from build123d import *

# Parameters (mm, degrees)
F1_DEPTH   = 762
F2_W       = 12.7
F2_H       = 25.4
F1_FACE1_W = 762
F1_FACE1_H = 7.0995158286
F3_DEPTH   = 38.101
F5_DEPTH   = 635.001
F7_DEPTH   = 635.001


# Not quite as in the source:
# - a feature names something its author has since deleted; it is built from what else it names


with BuildPart() as f1:
    # F0 (on Right) → F1 (new body)
    with BuildSketch(Plane.YZ):
        Polygon((-76.2, 6.35), (-127, -15.875), (-120.65, -19.05), (127, -19.05), (-25.4, 19.05), align=None)
    extrude(amount=F1_DEPTH)

    # F2 (on face) + F1_face1 (on face) → F3 (cut, through all)
    with BuildSketch(Plane(origin=(0, 0, -19.05), x_dir=(1, 0, 0), z_dir=(0, 0, -1))):
        Polygon((0, 120.65), (0, -127), (76.2, -127), (76.2, -76.2), (381, -76.2), (393.7, -76.2), (406.4, -76.2), (711.2, -76.2), (711.2, -127), (762, -127), (762, 120.65), align=None)
        with Locations((387.35, -88.9)):
            Rectangle(F2_W, F2_H)
        with Locations((400.05, -88.9)):
            Rectangle(F2_W, F2_H)
    with BuildSketch(Plane(origin=(381, -123.825, -17.4625), x_dir=(1, 0, 0), z_dir=(0, -0.4472135955, -0.894427191))):
        Rectangle(F1_FACE1_W, F1_FACE1_H)
    extrude(amount=-F3_DEPTH, dir=(0, 0, -1), mode=Mode.SUBTRACT)

    # F4 (on face) → F5 (cut, through all)
    with BuildSketch(Plane(origin=(76.2, 0, 0), x_dir=(0, -1, 0), z_dir=(-1, 0, 0))):
        Polygon((-76.2, -6.35), (-82.55, -7.9375), (-76.2, -15.875), align=None)
        Polygon((-76.2, -15.875), (-82.55, -19.05), (-76.2, -19.05), align=None)
    extrude(amount=-F5_DEPTH, mode=Mode.SUBTRACT)

    # F6 (on face) → F7 (cut, through all)
    with BuildSketch(Plane(origin=(76.2, 0, 0), x_dir=(0, -1, 0), z_dir=(-1, 0, 0))):
        with BuildLine():
            ThreePointArc((-82.55, -17.4625), (-81.4274679849, -16.9975320151), (-80.9625, -15.875))
            ThreePointArc((-80.9625, -15.875), (-83.6725320151, -14.7524679849), (-82.55, -17.4625))
        make_face()
    extrude(amount=-F7_DEPTH, mode=Mode.SUBTRACT)


solid = f1.part
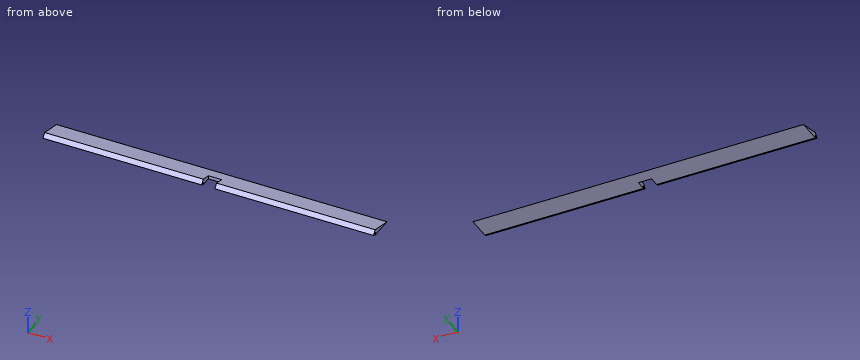
Build history of the part. All positions in model axes, mm. Round coordinates to 2 decimals unless told otherwise and drop trailing zeros. Loops run counter-clockwise (first coordinate to the right, second up) from the corner with the lowest first, then second, coordinate; pieces in that order, holes last. Notation, with made-up numbers: (-22.5, 32) -> (-3.5, 32) arc R10 ccw to (-3.5, 38) -> close; hole circle Ø10 at (-31.75, 44). An arc over 180 degrees is marked (long way). Use CSV: the item, a comma, the result in double quotes. Start each with the question number.
Q1. Flat gauge pins, fed straight in: pin 1 Ø3 at (x, z) = (393, -16.5) entering from -Y; pin 2 Ø5 at (y, z) = (94, -10) entering from +X; pin 3 Ø5 at (x, z) = (199, -12) entering from -Y; pin 4 Ø6 at (x, y) = (607.5, 84.5) entering from +Z. Where does each tip first touch, or does it go through?
Q2. Drill centre lines: L1, parallel to Z at x = 271, y = 83; L2, parallel to X at y = 90, z = -13; L3, parallel to Z at x = 202.5, y = 82.55. Where is each one in solid material? Low to high.
Q3. Saw through at A-A on z = -11. Give the cut face in (x, y), and give its area (3 significant figures).
Q4. Saw through at C-C on y = 113. Give the cut face in (x, z), and give its area (3 significant figures).
Solutions:
1,pin 1,"stops at y = 101.6"
1,pin 2,"stops at x = 711.2"
1,pin 3,"stops at y = 77.3"
1,pin 4,"stops at z = -7.94"
2,L1,"z = -19.05 to -17.4, -14.35 to -8.05"
2,L2,"x = 76.2 to 381, 406.4 to 711.2"
2,L3,"z = -19.05 to -17.46, -14.29 to -7.94"
3,outline,"(76.2, 80.1) -> (381, 80.1) -> (381, 94.8) -> (76.2, 94.8) -> close; (406.4, 80.1) -> (711.2, 80.1) -> (711.2, 94.8) -> (406.4, 94.8) -> close"
3,area,"8,960 mm^2"
4,outline,"(76.2, -19.05) -> (711.2, -19.05) -> (711.2, -15.55) -> (76.2, -15.55) -> close"
4,area,"2,220 mm^2"
